```python
from build123d import *

# Parameters (mm, degrees)
SKETCH1_R           = 35
BOSS_EXTRUDE1_DEPTH = 50
SKETCH6_R           = 25
BOSS_EXTRUDE2_DEPTH = 80
SKETCH7_R           = 35
BOSS_EXTRUDE3_DEPTH = 50
SKETCH10_R          = 30
BOSS_EXTRUDE5_DEPTH = 10
SKETCH12_W          = 70
SKETCH12_H          = 100.009163948
BOSS_EXTRUDE6_DEPTH = 50
CUT_EXTRUDE1_DEPTH  = 288.231322933
CUT_EXTRUDE2_DEPTH  = 281.761166962
FILLET1_R           = 15
SKETCH15_R          = 9
CUT_EXTRUDE3_DEPTH  = 288.208392811
BOSS_EXTRUDE8_DEPTH = 7.5
FILLET2_R           = 12
SKETCH17_R          = 6.5
CUT_EXTRUDE4_DEPTH  = 282.771025659
FILLET3_R           = 12
SKETCH18_W          = 15
SKETCH18_H          = 40
BOSS_EXTRUDE9_DEPTH = 50
CUT_EXTRUDE5_DEPTH  = 331.323570005
SKETCH20_R          = 11
CUT_EXTRUDE6_DEPTH  = 331.323570005


with BuildPart() as part:
    # Sketch1 → Boss-Extrude1 (new body)
    with BuildSketch(Plane(origin=(0, 0, 0), x_dir=(1, 0, 0), z_dir=(0, 1, 0))):
        with Locations(Location((0, 0, 0), (0, 0, 270))):
            Circle(SKETCH1_R)
    extrude(amount=BOSS_EXTRUDE1_DEPTH)

    # Sketch6 → Boss-Extrude2 (add)
    with BuildSketch(Plane(origin=(0, 50, 0), x_dir=(1, 0, 0), z_dir=(0, 1, 0))):
        with Locations(Location((0, 0, 0), (0, 0, 270))):
            Circle(SKETCH6_R)
    extrude(amount=BOSS_EXTRUDE2_DEPTH)

    # Sketch7 → Boss-Extrude3 (add)
    with BuildSketch(Plane(origin=(0, 130, 0), x_dir=(1, 0, 0), z_dir=(0, 1, 0))):
        with Locations(Location((0, 0, 0), (0, 0, 270))):
            Circle(SKETCH7_R)
    extrude(amount=BOSS_EXTRUDE3_DEPTH)



with BuildPart() as body_2:
    # Sketch10 → Boss-Extrude5 (new body)
    with BuildSketch(Plane(origin=(0, 250, 0), x_dir=(1, 0, 0), z_dir=(0, 1, 0))):
        with Locations(Location((0, 0, 0), (0, 0, 270))):
            Circle(SKETCH10_R)
    extrude(amount=BOSS_EXTRUDE5_DEPTH)


with BuildPart() as part_1:
    add(part.part)

    add(body_2.part)  # Revolve1 merges body 2
    # Sketch11 → Revolve1 (revolve)
    with BuildSketch(Plane(origin=(0, 0, 0), x_dir=(0, 0, -1), z_dir=(1, 0, 0))):
        Polygon((0, 250), (22.65711135, 250), (35, 180), (0, 180), align=None)
    revolve(axis=Axis((0, 180, 0), (0, 1, 0)))

    # Sketch12 → Boss-Extrude6 (add)
    with BuildSketch(Plane.XZ):
        with Locations((0, 50.004581974)):
            Rectangle(SKETCH12_W, SKETCH12_H)
    extrude(amount=-BOSS_EXTRUDE6_DEPTH)

    # Sketch13 → Cut-Extrude1 (cut, through all)
    with BuildSketch(Plane.ZY.offset(35)):
        Polygon((57.164723746, 50), (100.009163948, 20), (100.009163948, 50), align=None)
    extrude(amount=-CUT_EXTRUDE1_DEPTH, mode=Mode.SUBTRACT)

    # Sketch14 → Cut-Extrude2 (cut, through all)
    with BuildSketch(Plane.XZ):
        with BuildLine():
            Line((-20, 108.740570097), (20, 108.740570097))
            Line((20, 108.740570097), (20, 28.722813233))
            ThreePointArc((20, 28.722813233), (0, 35), (-20, 28.722813233))
            Line((-20, 28.722813233), (-20, 108.740570097))
        make_face()
    extrude(amount=-CUT_EXTRUDE2_DEPTH, mode=Mode.SUBTRACT)

    # Fillet1
    # the kernel refuses this fillet: 15 mm, written as the material it takes off along each edge
    with BuildSketch(Plane(origin=(-17.5, 0, 100.009163948), x_dir=(0, 0, -1), z_dir=(1, 0, 0)), Plane(origin=(-72.5, 0, 100.009163948), x_dir=(0, 0, -1), z_dir=(1, 0, 0))) as fillet1_piece_1:
        with BuildLine():
            CenterArc((FILLET1_R, FILLET1_R), FILLET1_R, 180, 90)
            Line((0, FILLET1_R), (0, 0))
            Line((0, 0), (FILLET1_R, 0))
        make_face()
    extrude(amount=90, mode=Mode.SUBTRACT)
    with BuildSketch(Plane(origin=(0.478735604, 20, 100.009163948), x_dir=(0, -1, 0), z_dir=(1, 0, 0)), Plane(origin=(-54.521264396, 20, 100.009163948), x_dir=(0, -1, 0), z_dir=(1, 0, 0))) as fillet1_piece_2:
        with BuildLine():
            CenterArc((FILLET1_R * 0.520567050552, FILLET1_R), FILLET1_R, 215, 55)
            Line((-FILLET1_R * 0.298584993737, FILLET1_R * 0.426423563649), (0, 0))
            Line((0, 0), (FILLET1_R * 0.520567050552, 0))
        make_face()
    extrude(amount=54.042528791, mode=Mode.SUBTRACT)

    # Sketch15 → Cut-Extrude3 (cut, through all)
    with BuildSketch(Plane.ZY.offset(35)):
        with Locations((67.943288424, 19)):
            Circle(SKETCH15_R)
    extrude(amount=-CUT_EXTRUDE3_DEPTH, mode=Mode.SUBTRACT)

    # Sketch16 → Boss-Extrude8 (add, symmetric)
    with BuildSketch(Plane(origin=(0, 0, 0), x_dir=(0, 0, -1), z_dir=(1, 0, 0))):
        Polygon((-35, 180), (-75, 155.965575239), (-75, 140), (-35, 140), (0, 140), (0, 180), align=None)
    boss_extrude8 = extrude(amount=BOSS_EXTRUDE8_DEPTH, both=True)

    # Fillet2
    # the kernel refuses this fillet: 12 mm, written as the material it takes off along each edge
    with BuildSketch(Plane(origin=(-37.5, 140, 75), x_dir=(0, 0, -1), z_dir=(1, 0, 0))) as fillet2_piece_1:
        with BuildLine():
            CenterArc((FILLET2_R, FILLET2_R), FILLET2_R, 180, 90)
            Line((0, FILLET2_R), (0, 0))
            Line((0, 0), (FILLET2_R, 0))
        make_face()
    extrude(amount=75, mode=Mode.SUBTRACT)
    with BuildSketch(Plane(origin=(-24.473183346, 155.965575239, 75), x_dir=(0, 0.5150380749100483, -0.8571673007021159), z_dir=(1, 0, 0))) as fillet2_piece_2:
        with BuildLine():
            CenterArc((FILLET2_R * 0.565772778188, -FILLET2_R), FILLET2_R, 90, 59)
            Line((-FILLET2_R * 0.291394522514, -FILLET2_R * 0.48496192509), (0, 0))
            Line((0, 0), (FILLET2_R * 0.565772778188, 0))
        make_face()
    extrude(amount=48.946366691, mode=Mode.SUBTRACT)

    # Sketch17 → Cut-Extrude4 (cut, through all)
    with BuildSketch(Plane(origin=(7.5, 0, 0), x_dir=(0, 0, -1), z_dir=(1, 0, 0))):
        with Locations((-55, 154.29)):
            Circle(SKETCH17_R)
    cut_extrude4 = extrude(amount=-CUT_EXTRUDE4_DEPTH, mode=Mode.SUBTRACT)

    # Mirror1: Boss-Extrude8 across plane
    add(boss_extrude8.mirror(Plane.XY))

    # Fillet3
    # the kernel refuses this fillet: 12 mm, written as the material it takes off along each edge
    with BuildSketch(Plane(origin=(-37.5, 140, -75), x_dir=(0, 0, 1), z_dir=(1, 0, 0))) as fillet3_piece_1:
        with BuildLine():
            CenterArc((FILLET3_R, -FILLET3_R), FILLET3_R, 90, 90)
            Line((0, -FILLET3_R), (0, 0))
            Line((0, 0), (FILLET3_R, 0))
        make_face()
    extrude(amount=75, mode=Mode.SUBTRACT)
    with BuildSketch(Plane(origin=(-24.473183346, 155.965575239, -75), x_dir=(0, 0.5150380749100483, 0.8571673007021159), z_dir=(1, 0, 0))) as fillet3_piece_2:
        with BuildLine():
            CenterArc((FILLET3_R * 0.565772778188, FILLET3_R), FILLET3_R, 211, 59)
            Line((-FILLET3_R * 0.291394522514, FILLET3_R * 0.48496192509), (0, 0))
            Line((0, 0), (FILLET3_R * 0.565772778188, 0))
        make_face()
    extrude(amount=48.946366691, mode=Mode.SUBTRACT)

    # Mirror2: Cut-Extrude4 across plane
    add(cut_extrude4.mirror(Plane.XY), mode=Mode.SUBTRACT)

    # Sketch18 → Boss-Extrude9 (add)
    with BuildSketch(Plane(origin=(0, 260, 0), x_dir=(1, 0, 0), z_dir=(0, 1, 0))):
        with Locations((-12.5, 0)):
            Rectangle(SKETCH18_W, SKETCH18_H)
    extrude(amount=BOSS_EXTRUDE9_DEPTH)

    # Sketch19 → Cut-Extrude5 (cut, through all)
    with BuildSketch(Plane.ZY.offset(20)):
        with BuildLine():
            Line((20, 310), (-1.45e-07, 310))
            ThreePointArc((-1.45e-07, 310), (14.142135572, 304.142135675), (20, 290))
            Line((20, 290), (20, 310))
        make_face()
        with BuildLine():
            Line((-20, 310), (-20, 290))
            ThreePointArc((-20, 290), (-14.142135675, 304.142135572), (-1.45e-07, 310))
            Line((-1.45e-07, 310), (-20, 310))
        make_face()
    extrude(amount=-CUT_EXTRUDE5_DEPTH, mode=Mode.SUBTRACT)

    # Sketch20 → Cut-Extrude6 (cut, through all)
    with BuildSketch(Plane.ZY.offset(20)):
        with Locations((0, 292.448780647)):
            Circle(SKETCH20_R)
    extrude(amount=-CUT_EXTRUDE6_DEPTH, mode=Mode.SUBTRACT)


solid = part_1.part
```
Read the model definition and answer for the solid it produces. Units are mm, in the model's axes. A direction names the side the tool comes from. Coordinates: 2 decimals unless noted, no trailing zeros. Loops run counter-clockwise (first coordinate to the right, second up) from the corner with the lowest first, then second, coordinate; pieces in that order, holes last. Notation, with made-up numbers: (83.25, 3) - (117.25, 3) arc R19 ccw to (117.25, 21) - close; hole circle Ø1 at (3.25, 81). An arc over 180 degrees is marked (long way). Answer in a Markdown table with one row per item.
1. Which of the six approach directions +Z, -Z, +X, -X, +Y, -Y give full straight-line access (tool end or side, diameter ignored) to faces 1 (the face through (-7.5, 160, -50)), 2 (the face through (26.89, 222.29, 5.97)), 3 (the face through (-7.5, 160, 50))?
Conclusion:
| item | result |
|---|---|
| face 1 | -Z, -X, +Y, -Y |
| face 2 | none |
| face 3 | +Z, -X, +Y, -Y |
2. Given pin 1 (3 mm diameter, centred on x = -8.5, y = 135.5, fed in from +Z); pin 2 (1 mm diameter, centred on x = 0, y = 105, fed in from +Z); pin 3 (12 mm diameter, centred on y = 155, z = 56, fed in from -X), each flat-ended and moving along its own axis, determine where each tip first touches the part or whether it passes through.
Conclusion:
| item | result |
|---|---|
| pin 1 | stops at z = 34.29 |
| pin 2 | stops at z = 25 |
| pin 3 | stops at x = -7.5 |
3. Find section D-D, the plane y = 211.5. Write down the section's boundary in (x, z), then the cut area to 3 significant figures.
Conclusion:
| item | result |
|---|---|
| outline | circle Ø58.89 at (0, 0) |
| area | 2,720 mm² |
4. Straight lines are drawn through the part: line 1 (Z direction, x = 2, y = 154); line 2 (Y direction, x = -14.5, z = 0); line 3 (Y direction, x = -4, z = -56). For each, find the intervals that lie inside material, in ascending order.
Conclusion:
| item | result |
|---|---|
| line 1 | z = -73.99 to -61.49, -48.51 to 48.51, 61.49 to 73.99 |
| line 2 | y = 0 to 281.45, 303.45 to 310 |
| line 3 | y = 140 to 147.87, 160.71 to 167.38 |
5. Find section A-A, the plane z = -55. Write down the section's boundary in (x, y).
Conclusion:
| item | result |
|---|---|
| outline | (-7.5, 140) - (7.5, 140) - (7.5, 147.79) - (-7.5, 147.79) - close; (-7.5, 160.79) - (7.5, 160.79) - (7.5, 167.98) - (-7.5, 167.98) - close |
6. Find section B-B, the plane y = 19. Write down the section's boundary in (x, z).
Conclusion:
| item | result |
|---|---|
| outline | (-35, 0) arc R35 ccw to (35, 0) - (35, 58.94) - (20, 58.94) - (20, 28.72) arc R35 ccw to (-20, 28.72) - (-20, 58.94) - (-35, 58.94) - close; (-35, 76.94) - (-20, 76.94) - (-20, 98.37) - (-35, 98.37) - close; (20, 76.94) - (35, 76.94) - (35, 98.37) - (20, 98.37) - close |
7. Determine the mould class of faces 4 (the face through (0.105, 169.875, 51.851)), 5 (the face through (7.5, 160, -50)), 6 (the face through (-20, 279, 0)), 7 (the face through (20, 19, 57)) for opening direction X: +X half, -X half, draft (parallel to the pull), parting line (faces both ways), or undercut.
Conclusion:
| item | result |
|---|---|
| face 4 | draft |
| face 5 | +X half |
| face 6 | -X half |
| face 7 | undercut |
8. Find section C-C, the plane y = 102.5. Write down the section's boundary in (x, z), then the cut area to 3 significant figures.
Conclusion:
| item | result |
|---|---|
| outline | circle Ø50 at (0, 0) |
| area | 1,960 mm² |
